Can you work these out from the model? Positions are in its coordinate system, mm. A direction names the side the tool comes from. Round coordinates to 2 decimals unless told otherwise and drop trailing zeros. Loops run counter-clockwise (first coordinate to the right, second up) from the corner with the lowest first, then second, coordinate; pieces in that order, holes last. Notation, with made-up numbers: M -25,-7.75 L 1,-7.75 A24 cw 1,25.25 Z; hole C 54,-35.5 d2. An arc over 180 degrees is marked long. Return JSON: item names as keys, results as strings.
```python
from build123d import *

# Parameters (mm, degrees)
EXTRUDE039_DEPTH = 15
EXTRUDE038_DEPTH = 26.5


with BuildPart() as extrude039:
    # Sketch046 → Extrude039 (new body)
    with BuildSketch(Plane(origin=(-14, 0, 0), x_dir=(0, -1, 0), z_dir=(-1, 0, 0))):
        Polygon((0, 4), (0, -12), (-8, -20), (-41, -20), (-41, 4), align=None)
    extrude(amount=-EXTRUDE039_DEPTH)


with BuildPart() as cut009:
    # Sketch045 → Extrude038 (new body)
    with BuildSketch(Plane.XY.offset(-25.5)):
        Polygon((-11, -1), (-11, 35), (0, 35), (0, 36), (-12, 36), (-12, -1), align=None)
    extrude(amount=EXTRUDE038_DEPTH)

    # Cut009: cut Extrude039
    add(extrude039.part, mode=Mode.SUBTRACT)


solid = cut009.part
```
Q1. On a 3-axis mill with a long thin cutter (end or side, diameter ignored), from which of +Z, -Z, +X, -X, +Y, -Y can I reach the whole of each face in a straight line? I mean faces 1 (the flat face through (-11, 12.9, -20.2)), 2 (the flat face through (-11.4, 26.1, -20)), 3 (the flat face through (-11.5, -0.5, 1)). Say none if no direction works.
Results:
{"face 1": "+Z, -Z, +X, -Y", "face 2": "+Z, +X, -X, +Y", "face 3": "+Z, +X, -X, +Y, -Y"}
Q2. Suppose I cut it at A-A, the plane z = -8.5. Please give me the cut outline in (x, y), plus the area to 3 significant figures.
Results:
{"outline": "M -12,-1 L -11,-1 L -11,0 L -12,0 Z", "area": "1.00 mm2"}
Q3. If I drill on line 1 along Z through (x, y) = (-11.5, 20); line 2 along X through (y, z) = (5, -23), over which ranges is the centre line in solid material (lowest first)?
Results:
{"line 1": "z = -25.5 to -20", "line 2": "x = -12 to -11"}
Q4. Suppose I cut it at B-B, the plane y = 18. Please give me the cut outline in (x, z).
Results:
{"outline": "M -12,-25.5 L -11,-25.5 L -11,-20 L -12,-20 Z"}
Q5. I'm going to push flat-ended pins straight in: pin 1 Ø5 at (x, y) = (-10, 17) entering from -Z; pin 2 Ø1.6 at (x, z) = (-8, -23) entering from -Y; pin 3 Ø1.5 at (x, z) = (-8.5, -17.5) entering from +Y. Where does each tip first touch, or does it pass through?
Results:
{"pin 1": "stops at z = -25.5", "pin 2": "stops at y = 35", "pin 3": "passes through"}
